Could you check a few things on this model? Use its own coordinates, in mm. A direction names the side the tool comes from. Give positions to 0.01 mm unless a question says otherwise; leave off trailing zeros. Loops run counter-clockwise (first coordinate to the right, second up) from the corner with the lowest first, then second, coordinate; pieces in that order, holes last.
1. Imagine slicing it at A-A (x = 426.5). List the corners of the cut face in (y, z) for me, plus the area to 3 significant figures.
2. I need wall thicknesses on line 1 along Y through (x, z) = (42.5, 1.75); line 2 along Y through (x, z) = (516, 3.5); line 3 along Y through (x, z) = (501.5, 2.25). Which ranges of each line are inside material? Lowest first, please.
3. For P1, Ø3, axis at y = 6, z = 3.5, coming from the -X side; P2, Ø3, axis at x = 536, z = 2, coming from the -Y side; P3, Ø1.5, axis at x = 331.5, z = 1, coming from the -Y side; P4, Ø2, axis at x = 61, z = 3, coming from the -Y side, each with a flat end and sliding along its axis, tell me the tip position at first contact or that it passes through.
4. For faces 1 (the flat face through (72.93, 7.395, 3.204)), 2 (the flat face through (280, 30, 0)), which set-ups out of +Z, -Z, +X, -X, +Y, -Y let a thin tool reach every point of the face, with its end or its side?
5. Imagine slicing it at B-B (z = 3.5). Count the separate pieces of the cut face and the enclosed holes in it, plus the area to 3 significant figures.
6. Thinking about a two-plate mould opening in X: for faces 3 (the flat face through (494.93, 7.605, 3.204)), 4 (the flat face through (280, 30, 6.5)), which applies, +X half, -X half, draft (parallel to the pull), parting line (faces both ways), or undercut?
Autodesk Inventor part; units mm, degrees
ref_plane "YZ Plane" through (0, 0, 0) normal (1, 0, 0) x (0, 1, 0)
ref_plane "XZ Plane" through (0, 0, 0) normal (0, 1, 0) x (-1, 0, 0)
ref_plane "XY Plane" through (0, 0, 0) normal (0, 0, 1) x (1, 0, 0)
sketch "Sketch1" plane through (0, 0, 0) normal (0, 0, 1) x (1, 0, 0)
  line L0 (568, 44.5) -> (0, 44.5)
  line L1 (68, 0) -> (78, 15)
  line L2 (78, 15) -> (490, 15)
  line L3 (490, 15) -> (500, 0)
  line L4 (0, 0) -> (68, 0)
  line L5 (500, 0) -> (568, 0)
  line L6 (0, 30) -> (68, 30)
  line L7 (68, 30) -> (68, 23.5)
  line L8 (68, 23.5) -> (0, 23.5)
  line L9 (0, 44.5) -> (0, 30)
  line L10 (0, 23.5) -> (0, 0)
  line L11 (568, 30) -> (500, 30)
  line L12 (500, 30) -> (500, 23.5)
  line L13 (500, 23.5) -> (568, 23.5)
  line L14 (568, 0) -> (568, 23.5)
  line L15 (568, 30) -> (568, 44.5)
  dimension "d3" = 6.5
  dimension "d4" = 68
  dimension "d5" = 68
  dimension "d6" = 568
  dimension "d7" = 15
  dimension "d8" = 23.5
  dimension "d9" = 14.5
  dimension "d12" = 10
  dimension "d13" = 10
  dimension "d14" = 10
  dimension "d15" = 10
extrude "Extrusion1" add sketch "Sketch1" along normal blind 6.5
sketch "Sketch2" plane through (0, 0, 6.5) normal (0, 0, 1) x (1, 0, 0)
  line L0 (0, 0) -> (68, 0)
  line L1 (500, 0) -> (568, 0)
  line L2 (568, 0) -> (568, 23.5)
  line L3 (568, 30) -> (568, 44.5)
  line L4 (568, 44.5) -> (0, 44.5)
  line L5 (0, 44.5) -> (0, 30)
  line L6 (0, 23.5) -> (0, 0)
  line L7 (24, 0) -> (35, 0)
  line L8 (35, 0) -> (35, 9)
  line L9 (35, 9) -> (24, 9)
  line L10 (24, 9) -> (24, 0)
  circle A0 centre (42.5, 4.5) radius 2.25
  circle A1 centre (52.5, 3.901) radius 2.75
  circle A2 centre (62.5, 4.5) radius 2.25
  line L11 (544, 0) -> (533, 0)
  line L12 (533, 0) -> (533, 9)
  line L13 (533, 9) -> (544, 9)
  line L14 (544, 9) -> (544, 0)
  circle A3 centre (505.5, 4.5) radius 2.25
  circle A4 centre (515.5, 3.901) radius 2.75
  circle A5 centre (525.5, 4.5) radius 2.25
  line L15 (107.9, 44.5) -> (117.9, 44.5)
  line L16 (117.9, 44.5) -> (117.9, 40.5)
  line L17 (116.9, 39.5) -> (108.9, 39.5)
  line L18 (107.9, 40.5) -> (107.9, 44.5)
  line L19 (450.1, 44.5) -> (460.1, 44.5)
  line L20 (460.1, 44.5) -> (460.1, 40.5)
  line L21 (459.1, 39.5) -> (451.1, 39.5)
  line L22 (450.1, 40.5) -> (450.1, 44.5)
  arc A6 (107.9, 40.5) -> (108.9, 39.5) centre (108.9, 40.5) ccw
  arc A7 (116.9, 39.5) -> (117.9, 40.5) centre (116.9, 40.5) ccw
  arc A8 (450.1, 40.5) -> (451.1, 39.5) centre (451.1, 40.5) ccw
  arc A9 (459.1, 39.5) -> (460.1, 40.5) centre (459.1, 40.5) ccw
  circle A10 centre (29.5, 3.901) radius 7.5 construction
  point P0 (538.5, 9)
  point P1 (35, 4.5)
  point P2 (112.9, 39.5)
  point P3 (455.1, 39.5)
  dimension "d16" = 11
  dimension "d18" = 4.5
  dimension "d19" = 5.5
  dimension "d20" = 11
  dimension "d21" = 1
  dimension "d22" = 10
  dimension "d23" = 10
  dimension "d27" = 24
  dimension "d29" = 23
  dimension "d30" = 24
  dimension "d31" = 10
  dimension "d32" = 10
  dimension "d33" = 10
  dimension "d34" = 10
  dimension "d35" = 9
  dimension "d38" = 15
  dimension "d39" = 23
  dimension "d49" = 112.9
  dimension "d50" = 112.9
  dimension "d63" = 5
extrude "Extrusion2" cut sketch "Sketch2" against normal through all
chamfer "Chamfer1" distance 2 angle 45 4 edges at (0, 44.5, 3.25) (0, 0, 3.25) (568, 44.5, 3.25) (568, 0, 3.25)
sketch "Sketch3" plane through (0, 0, 6.5) normal (0, 0, 1) x (1, 0, 0)
  line L0 (568, 2) -> (568, 23.5)
  line L1 (0, 23.5) -> (0, 2)
  circle A0 centre (52.5, 3.901) radius 2.75
  circle A1 centre (10, 3.901) radius 2
  circle A2 centre (558, 3.901) radius 2
  point P0 (0, 0)
  dimension "d43" = 4
  dimension "d44" = 10
  dimension "d45" = 4
  dimension "d46" = 10
extrude "Extrusion3" cut sketch "Sketch3" against normal through all contours A1 | A2
sketch "Sketch4" plane through (0, 0, 6.5) normal (0, 0, 1) x (1, 0, 0)
  line L0 (568, 2) -> (568, 23.5)
  line L1 (0, 23.5) -> (0, 2)
  line L2 (2, 0) -> (24, 0)
  line L3 (35, 0) -> (68, 0)
  line L4 (500, 0) -> (533, 0)
  line L5 (544, 0) -> (566, 0)
  line L6 (10, 0) -> (18, 0)
  line L7 (18, 0) -> (18, -6)
  line L8 (16, -8) -> (12, -8)
  line L9 (10, -6) -> (10, 0)
  line L10 (48.5, 0) -> (56.5, 0)
  line L11 (56.5, 0) -> (56.5, -6)
  line L12 (54.5, -8) -> (50.5, -8)
  line L13 (48.5, -6) -> (48.5, 0)
  line L14 (511.5, 0) -> (519.5, 0)
  line L15 (519.5, 0) -> (519.5, -6)
  line L16 (517.5, -8) -> (513.5, -8)
  line L17 (511.5, -6) -> (511.5, 0)
  line L18 (550, 0) -> (558, 0)
  line L19 (558, 0) -> (558, -6)
  line L20 (556, -8) -> (552, -8)
  line L21 (550, -6) -> (550, 0)
  arc A0 (10, -6) -> (12, -8) centre (12, -6) ccw
  arc A1 (16, -8) -> (18, -6) centre (16, -6) ccw
  arc A2 (48.5, -6) -> (50.5, -8) centre (50.5, -6) ccw
  arc A3 (54.5, -8) -> (56.5, -6) centre (54.5, -6) ccw
  arc A4 (511.5, -6) -> (513.5, -8) centre (513.5, -6) ccw
  arc A5 (517.5, -8) -> (519.5, -6) centre (517.5, -6) ccw
  arc A6 (550, -6) -> (552, -8) centre (552, -6) ccw
  arc A7 (556, -8) -> (558, -6) centre (556, -6) ccw
  point P0 (0, 0)
  dimension "d51" = 2
  dimension "d52" = 8
  dimension "d53" = 8
  dimension "d54" = 8
  dimension "d55" = 8
  dimension "d56" = 8
  dimension "d57" = 10
  dimension "d58" = 30.5
  dimension "d59" = 10
  dimension "d60" = 30.5
extrude "Extrusion4" add sketch "Sketch4" against normal blind 6.5
equation "\"d5\" = d4"
equation "\"d20\" = d16"
equation "\"d23\" = d22"
equation "\"d30\" = d27"
equation "\"d45\" = d43"
equation "\"d46\" = d44"
equation "\"d59\" = d57"
equation "\"d60\" = d58"
properties part number "x_axis_chain_holder" material "Plywood, Finish"
Derived:
1. outline: (15, 0) - (44.5, 0) - (44.5, 6.5) - (15, 6.5) - close
1. area: 192 mm2
2. line 1: y = 0 to 2.25, 6.75 to 23.5, 30 to 44.5
2. line 2: y = -8 to 1.2, 6.61 to 23.5, 30 to 44.5
2. line 3: y = 0 to 23.5, 30 to 44.5
3. P1: stops at x = 0
3. P2: stops at y = 9
3. P3: stops at y = 15
3. P4: stops at y = 0
4. face 1: +Z, -Z, -Y
4. face 2: -Z, +X, -X, +Y, -Y
5. separate pieces: 1
5. enclosed holes: 8
5. area: 17,900 mm2
6. face 3: undercut
6. face 4: draft
